from build123d import *

# Parameters (mm, degrees)
F0_R      = 22.8092
F1_DEPTH  = 27.432
F3_DEPTH  = 14.986
F4_R      = 19.05
F5_DEPTH  = 21.082
F8_D      = 5.1054
F8_DEPTH  = 7.5692
F8_START  = 0.1432934
F8_TIP    = 1.5338169022
F12_D     = 5.1054
F12_DEPTH = 3.7592
F12_START = 0.1432934
F12_TIP   = 1.5338169022


with BuildPart() as f1:
    # F0 (on Front) → F1 (new body)
    with BuildSketch(Plane.XZ):
        Circle(F0_R)
    extrude(amount=F1_DEPTH)

    # F2 (on face) → F3 (join)
    with BuildSketch(Plane(origin=(0, 0, 0), x_dir=(-1, 0, 0), z_dir=(0, 1, 0))):
        with BuildLine():
            Line((0, -4.0005), (2.5840677236, -4.0005))
            ThreePointArc((2.5840677236, -4.0005), (0, 4.7625), (-2.5840677236, -4.0005))
            Line((-2.5840677236, -4.0005), (0, -4.0005))
        make_face()
    extrude(amount=F3_DEPTH)

    # F4 (on face) → F5 (cut)
    with BuildSketch(Plane.XZ.offset(27.432)):
        Circle(F4_R)
    extrude(amount=-F5_DEPTH, mode=Mode.SUBTRACT)

    # F8
    # its depths count from where the whole tool has entered the part; down to there all is cleared
    with Locations(Plane(origin=(0, 0, -22.8092), x_dir=(1, 0, 0), z_dir=(0, 0, -1)).offset(-F8_START)):
        with Locations((0, 18.542)):
            Hole(F8_D / 2, depth=F8_DEPTH)
            with Locations((0, 0, -(F8_DEPTH + F8_TIP / 2))):  # 118° drill point
                Cone(0, F8_D / 2, F8_TIP, mode=Mode.SUBTRACT)

    # F12
    # its depths count from where the whole tool has entered the part; down to there all is cleared
    with Locations(Plane(origin=(19.75334664, 0, -11.4046), x_dir=(0, 1, 0), z_dir=(0.8660254038, 0, -0.5)).offset(-F12_START)):
        with Locations((-18.542, 0)):
            Hole(F12_D / 2, depth=F12_DEPTH)
            with Locations((0, 0, -(F12_DEPTH + F12_TIP / 2))):  # 118° drill point
                Cone(0, F12_D / 2, F12_TIP, mode=Mode.SUBTRACT)


solid = f1.part
The model under review builds one solid part; all positions refer to its coordinate system, in mm. A direction names the side the tool comes from. Give positions to 0.01 mm unless a question says otherwise; leave off trailing zeros. Order: outer loops, then holes, each group sorted by start corner. A loop starts at its lowest first (then second) coordinate and runs counter-clockwise, first axis right, second up. Notation, with made-up numbers: M -22,68 L 14,68 A21 cw 14,76 Z; hole C 54,-39.75 d10. An arc over 180 degrees is marked long. Answer in a Markdown table with one row per item. Add a question column.
1. To check wall thickness, follow line 1 along Y through (x, z) = (0, -21.1); line 2 along Y through (x, z) = (-1, 0); line 3 along Y through (x, z) = (9, 12.5). State the ranges of each line that lie inside material, in increasing order.
2. For pin 1 Ø3 at (y, z) = (-22.5, 0.5) entering from +X; pin 2 Ø5 at (x, z) = (4.5, 10.5) entering from +Y; pin 3 Ø10 at (y, z) = (2.5, -14.5) entering from +X; pin 4 Ø2 at (y, z) = (9, -3.5) entering from +X, all flat-tipped, find the tip position at first contact; note any pin that passes through.
3. Machinability: for faces 1 (the cylindrical face through (18.1, -15.99, -10.32)), 2 (the flat face through (0, -6.35, 0)), 3 (the cylindrical face through (0.332, -21.073, -20.817)), which of the approach directions +Z, -Z, +X, -X, +Y, -Y give a long, thin tool a straight path to every point of the face, cutting with its end or side? Answer none if there is none.
4. Add section D-D on y = -1.5. State the section outline as (x, z) points.
5. Add section C-C on x = -16.5. State the section outline as (y, z) points.
6. Mouldability with a two-part tool opening along X and no side actions: class faces 4 (the flat face through (0, 7, -4.001)), 5 (the cylindrical face through (-0.17, 7.39, 4.76)), 6 (the cylindrical face through (-15.12, -17.04, -11.59)) as released by +X, released by -X, zero draft, split by the parting line, or undercut.
7. Add section B-B on z = 0. State the section outline as (x, y) points, plus the area to 3 significant figures.
8. Add section A-A on x = 0. State the section outline as (y, z) points.
The answers:
| question | item | result |
|---|---|---|
| 1 | line 1 | -27.43 to -21.09, -15.99 to 0 |
| 1 | line 2 | -6.35 to 14.99 |
| 1 | line 3 | -6.35 to 0 |
| 2 | pin 1 | x = 22.81 |
| 2 | pin 2 | y = 0 |
| 2 | pin 3 | x = 20.42 |
| 2 | pin 4 | x = 4.05 |
| 3 | face 1 | none |
| 3 | face 2 | -Y |
| 3 | face 3 | -Z |
| 4 | outline | C 0,0 d45.62 |
| 5 | outline | M -27.43,-15.75 L 0,-15.75 L 0,15.75 L -27.43,15.75 L -27.43,9.52 L -6.35,9.52 L -6.35,-9.52 L -27.43,-9.52 Z |
| 6 | face 4 | zero draft |
| 6 | face 5 | split by the parting line |
| 6 | face 6 | undercut |
| 7 | outline | M -22.81,-27.43 L -19.05,-27.43 L -19.05,-6.35 L 19.05,-6.35 L 19.05,-27.43 L 22.81,-27.43 L 22.81,0 L 4.76,0 L 4.76,14.99 L -4.76,14.99 L -4.76,0 L -22.81,0 Z |
| 7 | area | 591 mm2 |
| 8 | outline | M -27.43,-22.81 L -21.09,-22.81 L -21.09,-19.05 L -27.43,-19.05 Z; M -27.43,19.05 L -6.35,19.05 L -6.35,-19.05 L -15.99,-19.05 L -15.99,-22.81 L 0,-22.81 L 0,-4 L 14.99,-4 L 14.99,4.76 L 0,4.76 L 0,22.81 L -27.43,22.81 Z |
